```python
from build123d import *

# Parameters (mm, degrees)
F3_DEPTH    = 4
F4_S6_R     = 8.85
F4_T7_DEPTH = 16


# Not quite as in the source:
# - a fillet or chamfer that OpenCascade refuses, or shapes differently, is made with other operations: its cross-section is extruded or revolved along the edge and cut away or added


with BuildPart() as f1:
    # F0 (on Front) → F1 (revolve)
    with BuildSketch(Plane.XZ):
        with BuildLine():
            Line((-11.75, 2.5), (-11.75, 0))
            Line((-11.75, 0), (-10.45, 0))
            Line((-10.45, 0), (-10.45, 1.2))
            Line((-10.45, 1.2), (-8.85, 1.2))
            Line((-8.85, 1.2), (-8.85, 4.2))
            ThreePointArc((-8.85, 4.2), (-8.5510140246, 10.7185269337), (-7.6565668329, 17.1823145401))
            ThreePointArc((-7.6565668329, 17.1823145401), (-7.3127346822, 17.7688675244), (-6.6733265732, 18))
            Line((-6.6733265732, 18), (0, 18))
            Line((0, 18), (0, 20))
            Line((0, 20), (-8.1253765053, 20))
            ThreePointArc((-8.1253765053, 20), (-8.7852885229, 19.7513428838), (-9.117016902, 19.1290322581))
            ThreePointArc((-9.117016902, 19.1290322581), (-9.7790230738, 12.3288025935), (-10, 5.5))
            Line((-10, 5.5), (-10, 2.5))
            Line((-10, 2.5), (-11.75, 2.5))
        make_face()
    revolve(axis=Axis((0, 0, 19), (0, 0, -1)))

    # F2 (on face) → F3 (cut)
    with BuildSketch(Plane.XY.offset(20)):
        Polygon((4.0626882527, 7.0367824689), (0, 4.0626882527), (-4.0626882527, 7.0367824689), (-3.5183912345, 2.0313441263), (-8.1253765053, 0), (-3.5183912345, -2.0313441263), (-4.0626882527, -7.0367824689), (0, -4.0626882527), (4.0626882527, -7.0367824689), (3.5183912345, -2.0313441263), (8.1253765053, 0), (3.5183912345, 2.0313441263), align=None)
    extrude(amount=-F3_DEPTH, mode=Mode.SUBTRACT)

    # F4: chamfer of 2 on 1 edges, made by hand


with BuildPart() as f4_tool2:
    # F4_s3 → F4_t4 (revolve)
    with BuildSketch(Plane.XZ):
        Polygon((-10.45, -0.8), (-8.45, 1.2), (-10.45, 1.2), align=None)
    revolve(axis=Axis((0, 0, 1.2), (0, 0, -1)))

    split(bisect_by=Plane.XY, keep=Keep.TOP)

    # F4_s6 → F4_t7 (cut, symmetric)
    with BuildSketch(Plane.XY.offset(0.2)):
        Circle(F4_S6_R)
    extrude(amount=F4_T7_DEPTH, both=True, mode=Mode.SUBTRACT)


with BuildPart() as f1_1:
    add(f1.part)

    # F4_t1: union F4_tool2
    add(f4_tool2.part)


solid = f1_1.part
```
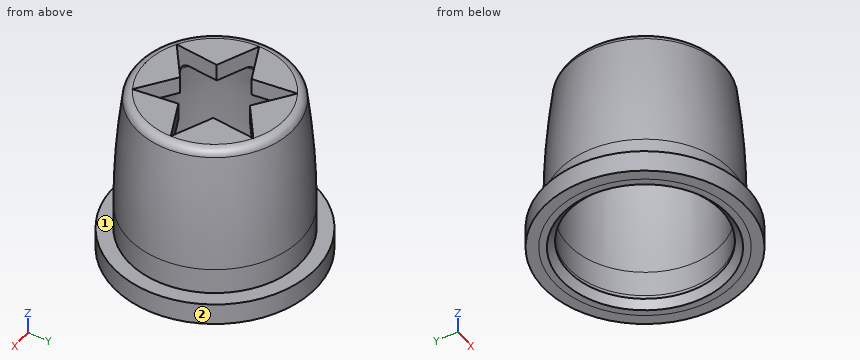
Can you work these out from the model? Positions are in its coordinate system, mm. Face numbers are marked on the shaded views. A direction names the side the tool comes from. Coordinates: 2 decimals unless noted, no trailing zeros. Write each loop counter-clockwise with the first axis right and the second up, starting at its lowest first coordinate (ties: lowest second). Pieces come first, ordered by that corner, then holes. Notation, with made-up numbers: (-13.5, 22) - (11.5, 22) arc R33 cw to (11.5, 52) - close; hole circle Ø3 at (54.5, -5). An arc over 180 degrees is marked (long way). Return JSON: item names as keys, results as strings.
Q1. I'm going to push flat-ended pins straight in: pin 1 Ø6 at (x, z) = (4.5, 7) entering from +Y; pin 2 Ø3 at (x, y) = (-1, -5) entering from -Z; pin 3 Ø2 at (x, y) = (0, 6) entering from -Z; pin 4 Ø1 at (x, y) = (-4, 1) entering from +Z. Where does each tip first touch, or does it pass through?
Computed values:
{"pin 1": "stops at y = 9.88", "pin 2": "stops at z = 18", "pin 3": "stops at z = 17.95", "pin 4": "passes through"}
Q2. If we section it at A-A (z = 3.75): Please give me the cut outline in (x, y).
Computed values:
{"outline": "circle Ø20 at (0, 0); hole circle Ø17.7 at (0, 0)"}
Q3. Please list where these lines run through material, in increasing order: L1, parallel to Y at x = 0, z = 3.2; L2, parallel to Y at x = 0, z = 1.8; L3, parallel to X at y = -3, z = 3. Write a range as from..to.
Computed values:
{"L1": "y = -10..-8.85, 8.85..10", "L2": "y = -11.75..-8.85, 8.85..11.75", "L3": "x = -9.54..-8.33, 8.33..9.54"}
Q4. On a 3-axis mill with a long thin cutter (end or side, diameter ignored), from which of +Z, -Z, +X, -X, +Y, -Y can I reach the whole of each face in a straight line? I mean the marked faces 1 and 2. Say none if no direction works.
Computed values:
{"face 1": "+Z", "face 2": "+Z, -Z"}
